Could you check a few things on this model? Use its own coordinates, in mm. A direction names the side the tool comes from. Coordinates: 2 decimals unless noted, no trailing zeros. Loops run counter-clockwise (first coordinate to the right, second up) from the corner with the lowest first, then second, coordinate; pieces in that order, holes last. Notation, with made-up numbers: (-12, -19.75) -> (22, -19.75) arc R14 ccw to (22, -2.75) -> close; hole circle Ø10 at (48, 10.25). An arc over 180 degrees is marked (long way). One line per question, with ' | ' between items.
```python
from build123d import *

# Parameters (mm, degrees)
SKETCH_1_R      = 5
SKETCH_1_R_2    = 2
SKETCH_1_R_3    = 2.08
SKETCH_1_R_4    = 8.75
EXTRUDE_1_DEPTH = 2


with BuildPart() as part:
    # 草图1 → 凸台-拉伸1 (new body)
    with BuildSketch(Plane.XY):
        with BuildLine():
            Line((341.797136251, -66.261433116), (-157.620006606, -66.261433116))
            ThreePointArc((-157.620006606, -66.261433116), (-176.265720892, -84.907147401), (-157.620006606, -103.552861687))
            Line((-157.620006606, -103.552861687), (341.797136251, -103.552861687))
            ThreePointArc((341.797136251, -103.552861687), (360.442850537, -84.907147401), (341.797136251, -66.261433116))
        make_face()
        with Locations((341.797136251, -84.907147401)):
            Circle(SKETCH_1_R, mode=Mode.SUBTRACT)
        with Locations((341.797136251, -69.907147401)):
            Circle(SKETCH_1_R_2, mode=Mode.SUBTRACT)
        with Locations((354.787517308, -92.261433116)):
            Circle(SKETCH_1_R_2, mode=Mode.SUBTRACT)
        with Locations((328.806755195, -92.407147401)):
            Circle(SKETCH_1_R_2, mode=Mode.SUBTRACT)
        with Locations((329.434548711, -77.769604157)):
            Circle(SKETCH_1_R_3, mode=Mode.SUBTRACT)
        with Locations((354.159723792, -77.623889871)):
            Circle(SKETCH_1_R_3, mode=Mode.SUBTRACT)
        with Locations((341.797136251, -99.036519604)):
            Circle(SKETCH_1_R_3, mode=Mode.SUBTRACT)
        with Locations((-157.620006606, -99.907147401)):
            Circle(SKETCH_1_R_2, mode=Mode.SUBTRACT)
        with Locations((-170.610387663, -92.407147401)):
            Circle(SKETCH_1_R_2, mode=Mode.SUBTRACT)
        with Locations((-170.610387663, -77.407147401)):
            Circle(SKETCH_1_R_2, mode=Mode.SUBTRACT)
        with Locations((-157.620006606, -69.907147401)):
            Circle(SKETCH_1_R_2, mode=Mode.SUBTRACT)
        with Locations((-144.629625549, -77.407147401)):
            Circle(SKETCH_1_R_2, mode=Mode.SUBTRACT)
        with Locations((-144.629625549, -92.407147401)):
            Circle(SKETCH_1_R_2, mode=Mode.SUBTRACT)
        with Locations((-171.150006606, -84.907147401)):
            Circle(SKETCH_1_R_3, mode=Mode.SUBTRACT)
        with Locations((-150.855006606, -73.189823688)):
            Circle(SKETCH_1_R_3, mode=Mode.SUBTRACT)
        with Locations((-150.855006606, -96.624471115)):
            Circle(SKETCH_1_R_3, mode=Mode.SUBTRACT)
        with Locations((-157.620006606, -84.907147401)):
            Circle(SKETCH_1_R_4, mode=Mode.SUBTRACT)
        with BuildLine():
            Line((-93.421962488, -75.424045387), (278.181949277, -75.424045387))
            ThreePointArc((278.181949277, -75.424045387), (287.665051291, -84.907147401), (278.181949277, -94.390249416))
            Line((278.181949277, -94.390249416), (-93.421962488, -94.390249416))
            ThreePointArc((-93.421962488, -94.390249416), (-102.905064503, -84.907147401), (-93.421962488, -75.424045387))
        make_face(mode=Mode.SUBTRACT)
    extrude(amount=EXTRUDE_1_DEPTH)


solid = part.part
```
Q1. For faces 1 (the face through (287.663, -84.699, 0.986)), 2 (the face through (88, -72, 0)), which set-ups out of +Z, -Z, +X, -X, +Y, -Y let a thin tool reach every point of the face, with its end or its side?
Values follow:
face 1: +Z, -Z | face 2: -Z, +X, -X, +Y, -Y
Q2. We'd pull the mould along X, two halves only. Please class faces 3 (the face through (-176.26, -84.5, 0.99)), 4 (the face through (-149.54, -88.26, 0.99)), 5 (the face through (88, -72, 2)), 6 (the face through (360.44, -85.32, 0.99)): released by +X, released by -X, zero draft, split by the parting line, or undercut.
Values follow:
face 3: released by -X | face 4: undercut | face 5: zero draft | face 6: released by +X
Q3. Imagine slicing it at A-A on x = 212.5. Write out the boundary of the cut face in (y, z).
Values follow:
outline: (-103.55, 0) -> (-94.39, 0) -> (-94.39, 2) -> (-103.55, 2) -> close; (-75.42, 0) -> (-66.26, 0) -> (-66.26, 2) -> (-75.42, 2) -> close
Q4. Please list where these lines run through material, in increasing order: L1, parallel to Y at x = 188, z = 0.5; L2, parallel to X at y = -71, z = 0.9 (3 decimals); L3, parallel to X at y = -68.5, z = 1. Write a range as [from, to].
Values follow:
L1: y = [-103.55, -94.39], [-75.42, -66.26] | L2: x = [-170.04, -159.295], [-155.945, 340.122], [343.472, 354.217] | L3: x = [-166.48, -159.04], [-156.2, 340.38], [343.22, 350.66]
Q5. For pin 1 (2.5 mm diameter, centred on x = 341.8, y = -99.04, fed in from +Z), with a flat end and sliding along its axis, tell me the tip position at first contact or that it passes through.
Values follow:
pin 1: passes through
Q6. Imagine slicing it at B-B on z = 1.6. Give the number of separate pieces and of enclosed holes in the cut face, plus the area to 3 significant figures.
Values follow:
separate pieces: 1 | enclosed holes: 18 | area: 11,900 mm2
